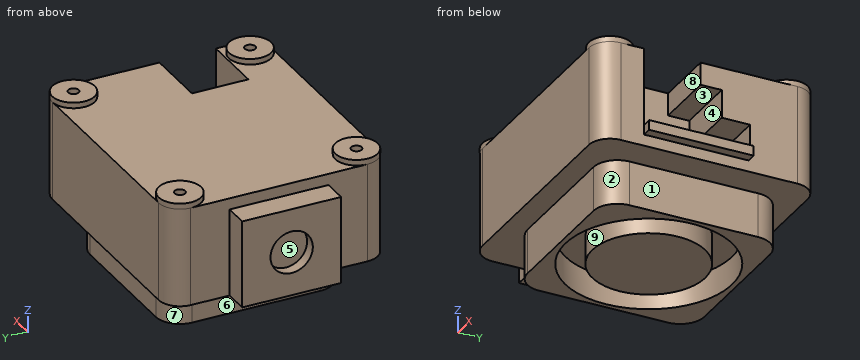
from build123d import *
from build123d.topology import SkipClean

# Parameters (mm, degrees)
BOSS_EXTRUDE1_DEPTH  = 14
SKETCH10_W           = 12.4
SKETCH10_H           = 14
BOSS_EXTRUDE5_DEPTH  = 3.5
SKETCH11_R           = 3
BOSS_EXTRUDE6_DEPTH  = 1.5
SKETCH11_2_R         = 3
CUT_EXTRUDE1_DEPTH   = 1.6
SKETCH12_W           = 3
SKETCH12_H           = 15
BOSS_EXTRUDE7_DEPTH  = 9
SKETCH13_W           = 3.2
SKETCH13_H           = 7
BOSS_EXTRUDE8_DEPTH  = 9
FILLET1_R            = 3
BOSS_EXTRUDE10_START = 0.8
SKETCH15_R           = 3
BOSS_EXTRUDE10_DEPTH = 0.8
SKETCH16_R           = 0.75
CUT_EXTRUDE2_DEPTH   = 5
SKETCH17_W           = 4
SKETCH17_H           = 4
BOSS_EXTRUDE11_DEPTH = 9
BOSS_EXTRUDE12_DEPTH = 6.3
SKETCH19_R           = 11.8
CUT_EXTRUDE3_DEPTH   = 4
SKETCH20_R           = 8
BOSS_EXTRUDE13_DEPTH = 4
SKETCH23_W           = 1.4
SKETCH23_H           = 14.8
BOSS_EXTRUDE14_DEPTH = 1.4


with BuildPart() as part:
    # Sketch1 → Boss-Extrude1 (new body)
    with BuildSketch(Plane.XY):
        Polygon((0, 0), (35.5, 0), (35.5, 6.3), (26.5, 6.3), (26.5, 21.3), (35.5, 21.3), (35.5, 31), (0, 31), align=None)
    extrude(amount=BOSS_EXTRUDE1_DEPTH)

    # Sketch10 → Boss-Extrude5 (add)
    with BuildSketch(Plane.ZY):
        with Locations((6.2, 15.5)):
            Rectangle(SKETCH10_W, SKETCH10_H)
    extrude(amount=BOSS_EXTRUDE5_DEPTH)

    # Sketch11 → Boss-Extrude6 (add)
    with BuildSketch(Plane.ZY.offset(3.5)):
        with Locations((6.2, 15.5)):
            Circle(SKETCH11_R)
    extrude(amount=-BOSS_EXTRUDE6_DEPTH)

    # Sketch11_2 → Cut-Extrude1 (cut)
    with BuildSketch(Plane.ZY.offset(3.5)):
        with Locations(Location((6.2, 15.5, 0), (0, 0, 270))):
            Circle(SKETCH11_2_R)
    extrude(amount=-CUT_EXTRUDE1_DEPTH, mode=Mode.SUBTRACT)

    # Sketch12 → Boss-Extrude7 (add)
    with BuildSketch(Plane(origin=(26.5, 0, 0), x_dir=(0, 0, -1), z_dir=(1, 0, 0))):
        with Locations((-1.5, 13.8)):
            Rectangle(SKETCH12_W, SKETCH12_H)
    extrude(amount=BOSS_EXTRUDE7_DEPTH)

    # Sketch13 → Boss-Extrude8 (add)
    with BuildSketch(Plane(origin=(26.5, 0, 0), x_dir=(0, 0, -1), z_dir=(1, 0, 0))):
        with Locations((-12.4, 17.8)):
            Rectangle(SKETCH13_W, SKETCH13_H)
    extrude(amount=BOSS_EXTRUDE8_DEPTH)

    # Fillet1
    fillet1_edges = [part.edges().sort_by_distance(p)[0] for p in [
        (0, 31, 7),
        (35.5, 31, 7),
        (35.5, 0, 7),
        (0, 0, 7),
    ]]
    fillet(fillet1_edges, radius=FILLET1_R)

    # Sketch15 → Boss-Extrude10 (add)
    with SkipClean():  # the faces are left unmerged after this step: merging them gives an invalid solid
        with BuildSketch(Plane.XY.offset(14).offset(BOSS_EXTRUDE10_START)):
            with Locations((32.5, 3)):
                Circle(SKETCH15_R)
            with Locations(Location((3, 3, 0), (0, 0, 180))):
                Circle(SKETCH15_R)
            with Locations(Location((3, 28, 0), (0, 0, 180))):
                Circle(SKETCH15_R)
            with Locations(Location((32.5, 28, 0), (0, 0, 180))):
                Circle(SKETCH15_R)
        extrude(amount=-BOSS_EXTRUDE10_DEPTH)

    # Sketch16 → Cut-Extrude2 (cut)
    with SkipClean():  # the faces are left unmerged after this step: merging them gives an invalid solid
        with BuildSketch(Plane.XY.offset(14.8)):
            with Locations((3, 28)):
                Circle(SKETCH16_R)
            with Locations((3, 3)):
                Circle(SKETCH16_R)
            with Locations((32.5, 3)):
                Circle(SKETCH16_R)
            with Locations((32.5, 28)):
                Circle(SKETCH16_R)
        extrude(amount=-CUT_EXTRUDE2_DEPTH, mode=Mode.SUBTRACT)

    # Sketch17 → Boss-Extrude11 (add)
    with SkipClean():  # the faces are left unmerged after this step: merging them gives an invalid solid
        with BuildSketch(Plane(origin=(26.5, 0, 0), x_dir=(0, 0, -1), z_dir=(1, 0, 0))):
            with Locations((-8.8, 19.3)):
                Rectangle(SKETCH17_W, SKETCH17_H)
        extrude(amount=BOSS_EXTRUDE11_DEPTH)

    # Sketch18 → Boss-Extrude12 (add)
    with SkipClean():  # the faces are left unmerged after this step: merging them gives an invalid solid
        with BuildSketch(Plane(origin=(0, 0, 0), x_dir=(-1, 0, 0), z_dir=(0, 0, -1))):
            with BuildLine():
                Line((-9.386280913, 3.15), (-27.6, 3.15))
                ThreePointArc((-27.6, 3.15), (-30.004163056, 4.145836944), (-31, 6.55))
                Line((-31, 6.55), (-31, 24.75))
                ThreePointArc((-31, 24.75), (-30.004163056, 27.154163056), (-27.6, 28.15))
                Line((-27.6, 28.15), (-9.4, 28.15))
                ThreePointArc((-9.4, 28.15), (-6.995836944, 27.154163056), (-6, 24.75))
                Line((-6, 24.75), (-6, 6.536280913))
                ThreePointArc((-6, 6.536280913), (-6.991818716, 4.141818716), (-9.386280913, 3.15))
            make_face()
        extrude(amount=BOSS_EXTRUDE12_DEPTH)

    # Sketch19 → Cut-Extrude3 (cut)
    with SkipClean():  # the faces are left unmerged after this step: merging them gives an invalid solid
        with BuildSketch(Plane(origin=(0, 0, -6.3), x_dir=(-1, 0, 0), z_dir=(0, 0, -1))):
            with Locations((-18.5, 15.646570228)):
                Circle(SKETCH19_R)
        extrude(amount=-CUT_EXTRUDE3_DEPTH, mode=Mode.SUBTRACT)

    # Sketch20 → Boss-Extrude13 (add)
    with SkipClean():  # the faces are left unmerged after this step: merging them gives an invalid solid
        with BuildSketch(Plane(origin=(0, 0, -2.3), x_dir=(-1, 0, 0), z_dir=(0, 0, -1))):
            with Locations((-18.496570228, 15.65)):
                Circle(SKETCH20_R)
        extrude(amount=BOSS_EXTRUDE13_DEPTH)

    # Sketch23 → Boss-Extrude14 (add)
    with SkipClean():  # the faces are left unmerged after this step: merging them gives an invalid solid
        with BuildSketch(Plane(origin=(35.5, 0, 0), x_dir=(0, 0, -1), z_dir=(1, 0, 0))):
            with Locations((-2.3, 13.7)):
                Rectangle(SKETCH23_W, SKETCH23_H)
        extrude(amount=BOSS_EXTRUDE14_DEPTH)


solid = part.part
Work out the finished part from the listing and answer in its coordinate system (mm). Face numbers are marked on the shaded views. A direction names the side the tool comes from. Round coordinates to 2 decimals unless told otherwise and drop trailing zeros. Write each loop counter-clockwise with the first axis right and the second up, starting at its lowest first coordinate (ties: lowest second). Pieces come first, ordered by that corner, then holes. Notation, with made-up numbers: (41.5, 85.25) -> (49.5, 85.25) arc R23 cw to (49.5, 121.25) -> close; hole circle Ø1 at (70, 10.25). An arc over 180 degrees is marked (long way). Answer as CSV lines item,"result". Start each with the question number.
(1) Find the intervals of material crossed by probe 1 along Y at (x, z) = (32.5, 13.1); probe 2 along Y at (x, z) = (18.5, -4.2); probe 3 along Y at (x, z) = (22, -5), in increasing order.
(2) The part is cut by section A-A, the plane x = 18.5. Give the vertices of the cut face in (y, z).
(3) The part is cut by section D-D, the plane z = -1.75. Give the vertices of the cut face in (x, y).
(4) The part is cut by section C-C, the plane y = 12. Give the vertices of the cut face in (x, z).
(5) A tool of negligible diameter and unlimited length cuts with its end or side. For the marked faces 5, 6, 7, 8 and 9, from which of +Z, -Z, +X, -X, +Y, -Y can it reach the whole face along a straight path? Write none if from no direction.
(6) The mould has two halves that part along Y. Classify the marked faces 1, 2, 3 and 4: +Y half, -Y half, draft (parallel to the pull), parting line (faces both ways), or undercut.
(7) The part is cut by section B-B, the plane z = 0.5. Give the vertices of the cut face in (x, y).
(8) Each of these flat-tipped pins is pushed along its axis until it touches: pin 1 (1.5 mm diameter, centred on x = 29.5, y = 16, fed in from -Z); pin 2 (5 mm diameter, centred on y = 22.5, z = 8, fed in from +X); pin 3 (5 mm diameter, centred on x = 18.5, z = -4, fed in from +Y); pin 4 (1.6 mm diameter, centred on x = 32.5, y = 3, fed in from +Z). Where does it stop, or does it pass through?
Output values:
1,probe 1,"y = 0 to 2.25, 3.75 to 6.3, 14.3 to 27.25, 28.75 to 31"
1,probe 2,"y = 3.15 to 3.85, 7.65 to 23.65, 27.45 to 28.15"
1,probe 3,"y = 3.15 to 4.38, 8.46 to 22.84, 26.92 to 28.15"
2,outline,"(0, 0) -> (3.15, 0) -> (3.15, -6.3) -> (3.85, -6.3) -> (3.85, -2.3) -> (7.65, -2.3) -> (7.65, -6.3) -> (23.65, -6.3) -> (23.65, -2.3) -> (27.45, -2.3) -> (27.45, -6.3) -> (28.15, -6.3) -> (28.15, 0) -> (31, 0) -> (31, 14) -> (0, 14) -> close"
3,outline,"(6, 6.54) arc R3.39 ccw to (9.39, 3.15) -> (27.6, 3.15) arc R3.4 ccw to (31, 6.55) -> (31, 24.75) arc R3.4 ccw to (27.6, 28.15) -> (9.4, 28.15) arc R3.4 ccw to (6, 24.75) -> close"
4,outline,"(-3.5, 0) -> (6, 0) -> (6, -6.3) -> (7.28, -6.3) -> (7.28, -2.3) -> (11.38, -2.3) -> (11.38, -6.3) -> (25.62, -6.3) -> (25.62, -2.3) -> (29.72, -2.3) -> (29.72, -6.3) -> (31, -6.3) -> (31, 0) -> (35.5, 0) -> (35.5, 1.6) -> (36.9, 1.6) -> (36.9, 3) -> (26.5, 3) -> (26.5, 14) -> (0, 14) -> (0, 12.4) -> (-3.5, 12.4) -> close"
5,face 5,"-X"
5,face 6,"-Z, -X, +Y, -Y"
5,face 7,"-Z, -X, +Y"
5,face 8,"+Z, +X"
5,face 9,"-Z"
6,face 1,"draft"
6,face 2,"-Y half"
6,face 3,"undercut"
6,face 4,"undercut"
7,outline,"(-3.5, 8.5) -> (0, 8.5) -> (0, 3) arc R3 ccw to (3, 0) -> (32.5, 0) arc R3 ccw to (35.5, 3) -> (35.5, 28) arc R3 ccw to (32.5, 31) -> (3, 31) arc R3 ccw to (0, 28) -> (0, 22.5) -> (-3.5, 22.5) -> close"
8,pin 1,"stops at z = -2.3"
8,pin 2,"stops at x = 35.5"
8,pin 3,"stops at y = 28.15"
8,pin 4,"stops at z = 14.8"
